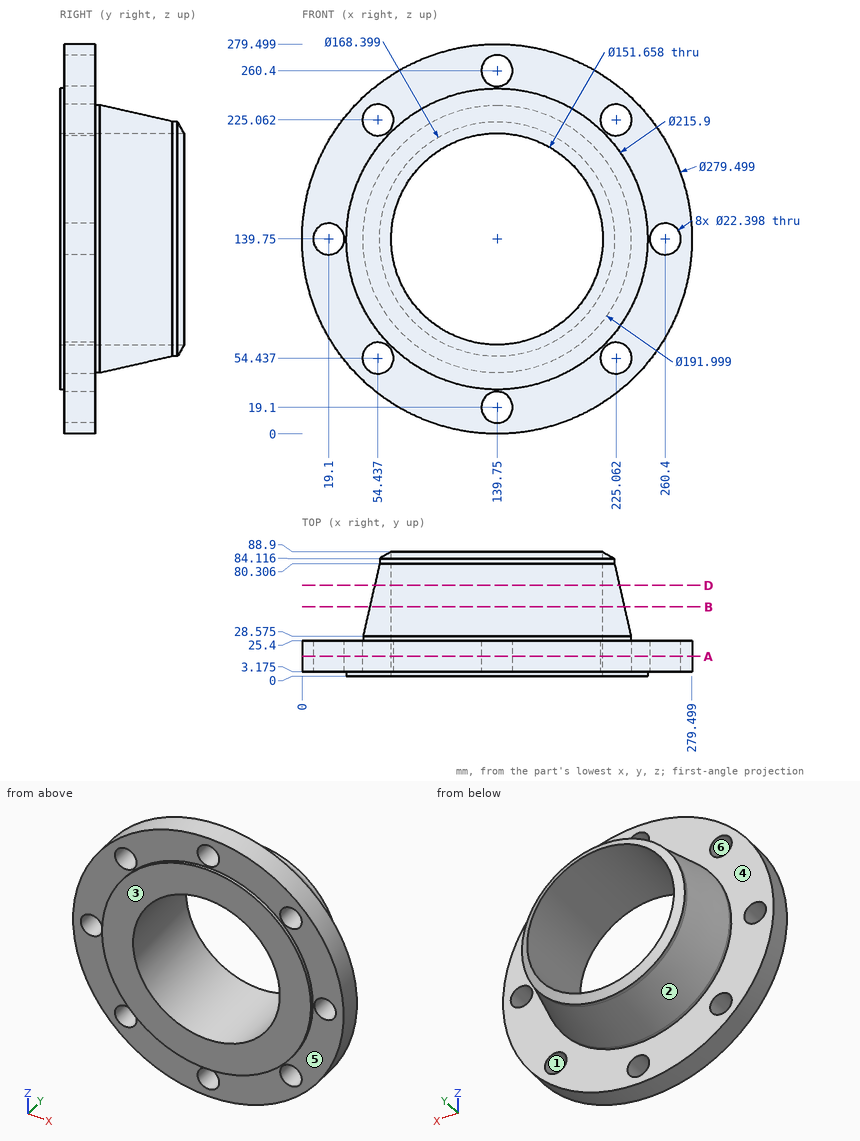
The figure shows three views and two pictorial views of one solid part (mm, origin at its lowest corner). Answer the questions. A direction names the side the tool comes from. Coordinates: 2 decimals unless noted, no trailing zeros. Loops run counter-clockwise (first coordinate to the right, second up) from the corner with the lowest first, then second, coordinate; pieces in that order, holes last. Notation, with made-up numbers: (48, -15.5) -> (52, -15.5) arc R4 ccw to (52, -9.5) -> close; hole circle Ø9 at (-35.75, -15). An arc over 180 degrees is marked (long way). Return JSON: item names as keys, results as strings. Group by question number.
(1) Which of the six approach directions +Z, -Z, +X, -X, +Y, -Y give full straight-line access (tool end or side, diameter ignored) to the marked faces 4, 5 and 6?
(2) A cutting plane is placed at D-D on y = 65. Write down the section's boundary in (x, z), and give its area (3 significant figures).
(3) A cutting plane is placed at A-A on y = 14. Count the separate pieces of the cut face and the enclosed holes in it, and give its area (3 significant figures).
(4) Determine the mould class of the marked faces 1, 2 and 3 for opening direction Z: released by +Z, released by -Z, zero draft, split by the parting line, or undercut.
(5) A cutting plane is placed at B-B on y = 49.5. Write down the section's boundary in (x, z), and give its area (3 significant figures).
(6) Find the intervals of material crossed by probe 1 along Y at (x, z) = (259, 114.5) (1 decimal); probe 2 along X at (y, z) = (47, 130); probe 3 along Z at (x, y) = (108, 19.5) (1 decimal), in increasing order. Write a range as from..to.
(7) Given pin 1 Ø2 at (y, z) = (40.5, 214.5) entering from +X (1 decimal); pin 2 Ø5 at (x, z) = (82.5, 250) entering from -Y (3 decimals); pin 3 Ø6 at (y, z) = (28, 207) entering from -X (1 decimal), each flat-ended and moving along its own axis, determine where each tip first touches the part or whether it passes through.
The answers:
{
 "1": {"face 4": "+Y", "face 5": "-Y", "face 6": "+Y, -Y"},
 "2": {"outline": "circle Ø175.38 at (139.75, 139.75); hole circle Ø151.66 at (139.75, 139.75)", "area": "6,090 mm^2"},
 "3": {"separate pieces": "1", "enclosed holes": "9", "area": "40,100 mm^2"},
 "4": {"face 1": "undercut", "face 2": "split by the parting line", "face 3": "zero draft"},
 "5": {"outline": "circle Ø182.45 at (139.75, 139.75); hole circle Ø151.66 at (139.75, 139.75)", "area": "8,080 mm^2"},
 "6": {"probe 1": "y = 3.2..25.4", "probe 2": "x = 48.47..64.55, 214.95..231.03", "probe 3": "z = 3.7..70.9, 208.6..275.8"},
 "7": {"pin 1": "stops at x = 196.9", "pin 2": "stops at y = 3.175", "pin 3": "stops at x = 16.4"}
}
